Answer from the drawing. Dimensions are ordinates in mm from the lowest x, y and z of the part. Give positions to 0.01 mm unless a question says otherwise; leave off trailing zeros. Write each loop counter-clockwise with the first axis right and the second up, starting at its lowest first coordinate (ties: lowest second). Pieces come first, ordered by that corner, then holes. Notation, with made-up numbers: (25.25, 63) -> (43.25, 63) arc R33 cw to (43.25, 98) -> close; hole circle Ø10 at (63.5, 85). An arc over 180 degrees is marked (long way). Write item = value, one per line.
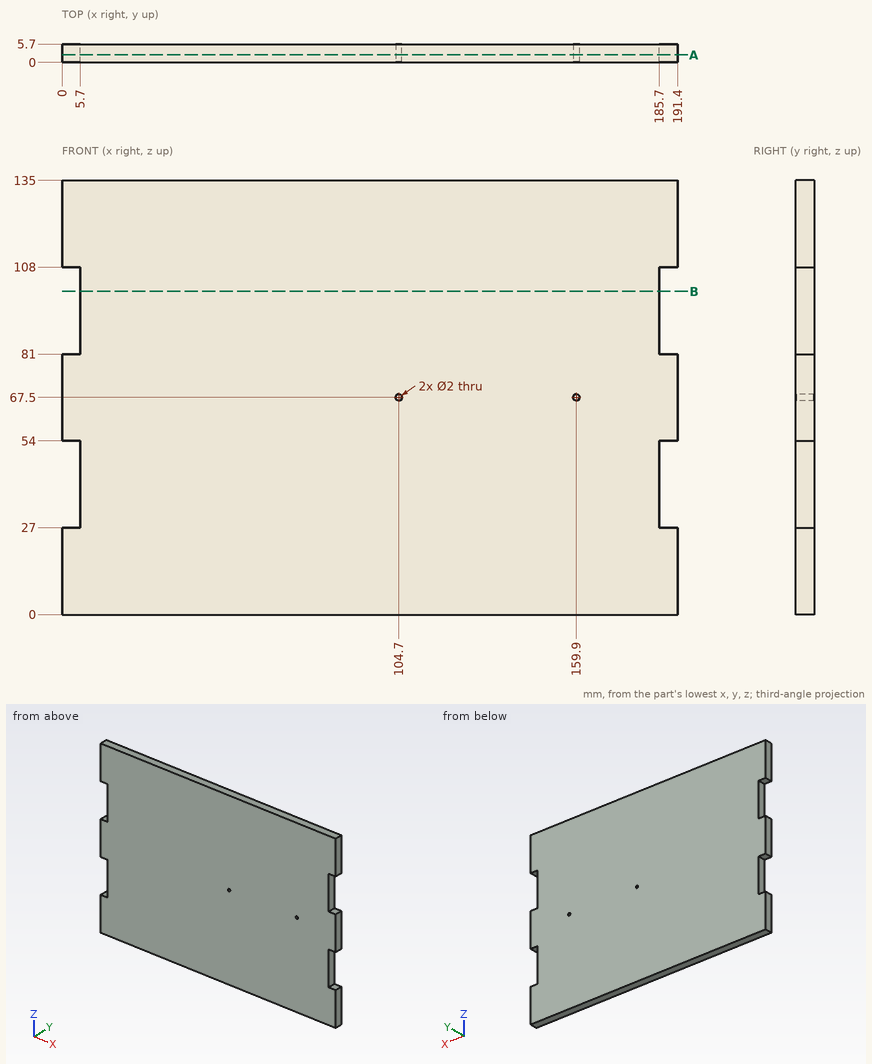
(1) Consider L1, parallel to X at y = 2.75, z = 67.5; L2, parallel to Z at x = 104.7, y = 4.1; L3, parallel to X at y = 1.8, z = 36. Determine where each line is inside the solid, lowest interval first.
Checks:
L1 = 0 to 103.7, 105.7 to 158.9, 160.9 to 191.4
L2 = 0 to 66.5, 68.5 to 135
L3 = 5.7 to 185.7
(2) The part is cut by section B-B on z = 100.5. Determine the outline of the cut face in (x, y), plus the area to 3 significant figures.
Checks:
outline = (5.7, 0) -> (185.7, 0) -> (185.7, 5.7) -> (5.7, 5.7) -> close
area = 1,030 mm²
(3) The part is cut by section A-A on y = 2.3. Determine the outline of the cut face in (x, z), plus the area to 3 significant figures.
Checks:
outline = (0, 0) -> (191.4, 0) -> (191.4, 27) -> (185.7, 27) -> (185.7, 54) -> (191.4, 54) -> (191.4, 81) -> (185.7, 81) -> (185.7, 108) -> (191.4, 108) -> (191.4, 135) -> (0, 135) -> (0, 108) -> (5.7, 108) -> (5.7, 81) -> (0, 81) -> (0, 54) -> (5.7, 54) -> (5.7, 27) -> (0, 27) -> close; hole circle Ø2 at (104.7, 67.5); hole circle Ø2 at (159.9, 67.5)
area = 25,200 mm²
(4) Given P1, Ø3, axis at y = 4, z = 95.5, coming from the -X side; P2, Ø1, axis at x = 164, y = 1.5, coming from the -Z side; P3, Ø3, axis at y = 3.5, z = 93, coming from the +X side, each flat-ended and moving along its own axis, determine where each tip first touches the part or whether it passes through.
Checks:
P1 = 5.7
P2 = 0
P3 = 185.7
